For this review, take the finished solid that the model builds, in its own axes (mm). A direction names the side the tool comes from. Round coordinates to 2 decimals unless told otherwise and drop trailing zeros. Write each loop counter-clockwise with the first axis right and the second up, starting at its lowest first coordinate (ties: lowest second). Pieces come first, ordered by that corner, then holes. Notation, with made-up numbers: (25, 49.25) -> (41, 49.25) arc R33 cw to (41, 87.25) -> close; hole circle Ø8 at (87.5, 44). An arc over 180 degrees is marked (long way). Write each question's results on one line, items separated by ' | '. Start each with the question number.
Item 1: Add section B-B (z = 0). State the section outline as (x, y) points.
Item 2: The part is to be moulded in two halves that separate along Z. For faces 3 (the cylindrical face through (-3.955, 1.972, -5.158)), 4 (the cylindrical face through (43.58, 2.46, 0.74)), 5 (the flat face through (-1, 2, 10)), 6 (the flat face through (-1, 5, -9)), say which applies: +Z half, -Z half, draft (parallel to the pull), parting line (faces both ways), or undercut.
Item 3: Clearance check with a flat-ended pin moving along its axis: pin 1 (10 mm diameter, centred on x = 29.5, z = 7.5, fed in from -Y). State where the tip first meets the part, or that it passes through.
Item 4: Add section C-C (y = 2.3). State the section outline as (x, z) points.
Item 5: Tool access review of faces 1 (the flat face through (3, 4, -6)), 2 (the cylindrical face through (-46.42, 2.46, 0.74)): name each direction out of +Z, -Z, +X, -X, +Y, -Y from which nothing blocks a thin tool from reaching the whole face with its end or side.
Item 6: To check wall thickness, follow line 1 along X through (y, z) = (3.95, 0); line 2 along X through (y, z) = (1, 5.5); line 3 along Z through (x, y) = (44, 3.95). State the ranges of each line that lie inside material, in increasing order.
Item 7: Add section A-A (x = 45). State the section outline as (y, z) points.
Item 8: Add section D-D (z = 4.75). State the section outline as (x, y) points, plus the area to 3 significant figures.
from build123d import *

# Parameters (mm, degrees)
SKETCH_1_W          = 100
SKETCH_1_H          = 20
SKETCH_1_R          = 1.6
SKETCH_1_R_2        = 6.5
EXTRUDE_1_DEPTH     = 5
SKETCH_2_R          = 7.5
CUT_EXTRUDE_1_DEPTH = 1


with BuildPart() as part:
    # 草图1 → 凸台-拉伸1 (new body)
    with BuildSketch(Plane(origin=(0, 0, 0), x_dir=(1, 0, 0), z_dir=(0, 1, 0))):
        Rectangle(SKETCH_1_W, SKETCH_1_H)
        with Locations(Location((45, 0, 0), (0, 0, 270))):
            Circle(SKETCH_1_R, mode=Mode.SUBTRACT)
        with Locations(Location((-45, 0, 0), (0, 0, 270))):
            Circle(SKETCH_1_R, mode=Mode.SUBTRACT)
        with Locations(Location((0, 0, 0), (0, 0, 270))):
            Circle(SKETCH_1_R_2, mode=Mode.SUBTRACT)
    extrude(amount=EXTRUDE_1_DEPTH)

    # 草图2 → 切除-拉伸1 (cut)
    with BuildSketch(Plane(origin=(0, 5, 0), x_dir=(1, 0, 0), z_dir=(0, 1, 0))):
        with Locations(Location((0, 0, 0), (0, 0, 270))):
            Circle(SKETCH_2_R)
    extrude(amount=-CUT_EXTRUDE_1_DEPTH, mode=Mode.SUBTRACT)


solid = part.part
Responses:
1) outline: (-50, 0) -> (-46.6, 0) -> (-46.6, 5) -> (-50, 5) -> close; (-43.4, 0) -> (-6.5, 0) -> (-6.5, 4) -> (-7.5, 4) -> (-7.5, 5) -> (-43.4, 5) -> close; (6.5, 0) -> (43.4, 0) -> (43.4, 5) -> (7.5, 5) -> (7.5, 4) -> (6.5, 4) -> close; (46.6, 0) -> (50, 0) -> (50, 5) -> (46.6, 5) -> close
2) face 3: undercut | face 4: undercut | face 5: +Z half | face 6: draft
3) pin 1: stops at y = 0
4) outline: (-50, -10) -> (50, -10) -> (50, 10) -> (-50, 10) -> close; hole circle Ø3.2 at (-45, 0); hole circle Ø13 at (0, 0); hole circle Ø3.2 at (45, 0)
5) face 1: +Y | face 2: +Y, -Y
6) line 1: x = -50 to -46.6, -43.4 to -6.5, 6.5 to 43.4, 46.6 to 50 | line 2: x = -50 to -3.46, 3.46 to 50 | line 3: z = -10 to -1.25, 1.25 to 10
7) outline: (0, -10) -> (5, -10) -> (5, -1.6) -> (0, -1.6) -> close; (0, 1.6) -> (5, 1.6) -> (5, 10) -> (0, 10) -> close
8) outline: (-50, 0) -> (-4.44, 0) -> (-4.44, 4) -> (-5.8, 4) -> (-5.8, 5) -> (-50, 5) -> close; (4.44, 0) -> (50, 0) -> (50, 5) -> (5.8, 5) -> (5.8, 4) -> (4.44, 4) -> close | area: 453 mm^2
